Geometry check sheet. Reference: the model listing, model coordinates, mm. Face numbers are marked on the shaded views. A direction names the side the tool comes from. Give positions to 0.01 mm unless a question says otherwise; leave off trailing zeros. Order: outer loops, then holes, each group sorted by start corner. A loop starts at its lowest first (then second) coordinate and runs counter-clockwise, first axis right, second up.
Autodesk Inventor part; units mm, degrees
ref_plane "YZ Plane" through (0, 0, 0) normal (1, 0, 0) x (0, 1, 0)
ref_plane "XZ Plane" through (0, 0, 0) normal (0, 1, 0) x (-1, 0, 0)
ref_plane "XY Plane" through (0, 0, 0) normal (0, 0, 1) x (1, 0, 0)
sketch "Sketch1" plane through (0, 0, 0) normal (0, 0, 1) x (1, 0, 0)
  circle A0 centre (0, 0) radius 1.5
  circle A1 centre (0, 0) radius 5
  dimension "d0" = 3
  dimension "d1" = 10
extrude "Extrusion1" add sketch "Sketch1" along normal blind 3
sketch "Sketch2" plane through (0, 0, 3) normal (0, 0, 1) x (1, 0, 0)
  circle A0 centre (0, 0) radius 5
  line L0 (4.7697, 1.5) -> (5.7697, 1.5)
  line L1 (5.7697, 1.5) -> (5.7697, -1.5)
  line L2 (5.7697, -1.5) -> (4.7697, -1.5)
  line L3 (4.7697, -1.5) -> (4.7697, 1.5)
  circle A1 centre (0, 0) radius 5
  point P0 (4.7697, 0)
  dimension "d4" = 1
  dimension "d8" = 3
extrude "Extrusion2" add sketch "Sketch2" against normal blind 3 contours A0 L3 | A0 L0 L1 L2 picked at (4.8122, -0.3362)
sketch "Sketch3" plane through (5.7697, -1.5, 3) normal (1, 0, 0) x (0, 0, -1)
  line L0 (-1.5, 4.5) -> (4.5, 4.5)
  line L1 (4.5, 4.5) -> (4.5, -1.5)
  line L2 (4.5, -1.5) -> (-1.5, -1.5)
  line L3 (-1.5, -1.5) -> (-1.5, 4.5)
  line L4 (0, 3) -> (3, 3)
  line L5 (0, 3) -> (0, 0)
  point P0 (3, 1.5)
  point P1 (0, 1.5)
  point P2 (-1.5, 1.5)
  point P3 (1.5, 3)
  point P4 (1.5, 4.5)
  dimension "d9" = 6
  dimension "d10" = 6
extrude "Extrusion3" add sketch "Sketch3" along normal blind 18
sketch "Sketch4" plane through (5.7697, -3, 4.5) normal (0, 0, 1) x (1, 0, 0)
  line L0 (18, 7.75) -> (18, -1.75)
  line L1 (18, 6) -> (18, 0)
  line L2 (0, 0) -> (0, 6)
  arc A0 (0, 6) -> (18, 7.75) centre (-5.4885, 155.8996) ccw
  arc A1 (18, -1.75) -> (0, 0) centre (-5.4885, -149.8996) ccw
  line L3 (0, 0) -> (18, 0)
  line L4 (0, 0) -> (18, 0)
  line L5 (18, 0) -> (18, -1.75)
  line L6 (0, 6) -> (18, 6)
  line L7 (0, 6) -> (18, 6)
  line L8 (18, 6) -> (18, 7.75)
  point P0 (-5.7697, 3)
  point P1 (18, 3)
  dimension "d13" = 9.5
  dimension "d14" = 150
  dimension "d15" = 150
extrude "Extrusion4" add sketch "Sketch4" against normal blind 6 contours L0 L6 A0 | L0 A1 L3
sketch "Sketch5" plane through (4.7697, 1.5, 3) normal (0, 1, 0) x (1, 0, 0)
  line L0 (19, 6.25) -> (19, -3.25)
  line L1 (19, -1.5) -> (19, 4.5)
  arc A0 (1, 4.5) -> (19, 6.25) centre (-4.4885, 154.3996) ccw
  line L2 (19, -1.5) -> (1, -1.5)
  arc A1 (19, -3.25) -> (1, -1.5) centre (-4.4885, -151.3996) ccw
  line L3 (1, 4.5) -> (19, 4.5)
  line L4 (19, 4.5) -> (19, 6.25)
  line L5 (1, -1.5) -> (19, -1.5)
  line L6 (19, -1.5) -> (19, -3.25)
  point P0 (-4.7697, 3)
  point P1 (19, 1.5)
  dimension "d18" = 9.5
  dimension "d19" = 150
  dimension "d20" = 150
extrude "Extrusion5" add sketch "Sketch5" along normal blind 3.25 and the other way blind 6.25
sketch "Sketch6" plane through (5.7697, -4.75, -1.5) normal (0, 0, 1) x (1, 0, 0)
  arc A0 (0, 7.75) -> (18, 9.5) centre (-5.4885, 157.6496) ccw
  line L0 (0, 9.5) -> (18, 9.5)
  line L1 (0, 7.75) -> (0, 9.5)
  arc A1 (18, 0) -> (0, 1.75) centre (-5.4885, -148.1496) ccw
  line L2 (0, 0) -> (0, 1.75)
  line L3 (18, 0) -> (0, 0)
  point P0 (-5.7697, 4.75)
extrude "Extrusion6" cut sketch "Sketch6" along normal through all both and the other way through all
fillet "Fillet1" radius 2 4 edges at (14.7961, 3.6035, -2.1035) (14.872, 3.6109, 5.1109) (14.872, -3.6109, 5.1109) (14.7961, -3.6035, -2.1035)
sketch "Sketch7" plane through (23.7697, -1.5, 3) normal (1, 0, 0) x (0, 0, -1)
  circle A0 centre (1.5, 1.5) radius 1.5
  line L0 (-3.25, 4.2747) -> (-3.25, -1.2747)
  line L1 (-1.2747, 6.25) -> (4.2747, 6.25)
  point P0 (3, 1.5)
  point P1 (1.5, 6.25)
  point P2 (-3.25, 1.5)
  dimension "d28" = 3
extrude "Extrusion7" cut sketch "Sketch7" against normal blind 10
properties part number "Arm4" material "ABS Plastic"
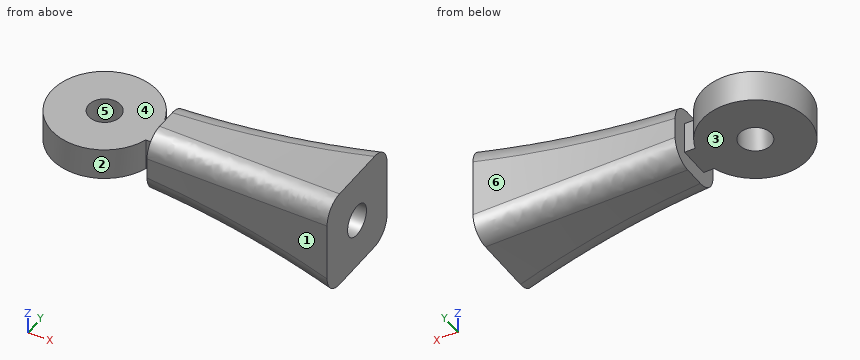
Item 1: Gauge pin test, flat ends, axial feed: pin 1 (2 mm diameter, centred on x = 12.5, z = -2, fed in from -Y); pin 2 (3 mm diameter, centred on x = 4, y = -3, fed in from -Z); pin 3 (4 mm diameter, centred on y = 0, z = 1.5, fed in from +X); pin 4 (0.8 mm diameter, centred on x = 5, z = 1, fed in from +Y). Record the tip position at first contact, or that the pin passes through.
Reported:
pin 1: stops at y = -3.09
pin 2: stops at z = 0
pin 3: stops at x = 23.77
pin 4: stops at y = 1.96
Item 2: Draft check along Y on the marked faces 4, 5 and 6. Enter one of: released by +Y, released by -Y, zero draft, split by the parting line, or undercut.
Reported:
face 4: zero draft
face 5: undercut
face 6: released by +Y
Item 3: Set-up check for the marked faces 1, 2 and 3: record each of +Z, -Z, +X, -X, +Y, -Y from which the full face is reachable in a straight line by a thin tool's end or side.
Reported:
face 1: +Z, -Z, -Y
face 2: +Z, -Z
face 3: -Z, -X, +Y, -Y
Item 4: Sectioned sample at C-C (z = 1.5). Enter the section's corners in (x, y).
Reported:
outline: (4.77, -1.5) - (5.77, -1.5) - (5.77, -3) arc R150 cw to (23.77, -4.75) - (23.77, -1.5) - (13.77, -1.5) - (13.77, 1.5) - (23.77, 1.5) - (23.77, 4.75) arc R150 cw to (5.77, 3) - (5.77, 1.5) - (4.77, 1.5) arc R5 ccw (long way) to start; hole circle Ø3 at (0, 0)
Item 5: Sectioned sample at A-A (y = 0). Enter the section's corners in (x, z).
Reported:
outline: (-5, 0) - (-1.5, 0) - (-1.5, 3) - (-5, 3) - close; (1.5, 0) - (5.77, 0) - (5.77, -1.5) arc R150 cw to (23.77, -3.25) - (23.77, 0) - (13.77, 0) - (13.77, 3) - (23.77, 3) - (23.77, 6.25) arc R150 cw to (5.77, 4.5) - (5.77, 3) - (1.5, 3) - close
Item 6: Sectioned sample at B-B (x = 0). Enter the section's corners in (y, z), and give its area (3 significant figures).
Reported:
outline: (-5, 0) - (-1.5, 0) - (-1.5, 3) - (-5, 3) - close; (1.5, 0) - (5, 0) - (5, 3) - (1.5, 3) - close
area: 21.0 mm2
Item 7: Scan lines: L1, parallel to Y at x = 0, z = 1.6; L2, parallel to X at y = -2.5, z = 1; L3, parallel to Y at x = 18.25, z = 1. Record each from-to range of solid material in increasing order.
Reported:
L1: y = -5 to -1.5, 1.5 to 5
L2: x = -4.33 to 4.33, 5.77 to 23.77
L3: y = -3.98 to -1.41, 1.41 to 3.98
